Design review of the part shown in the three views and the two pictorial views. Dimensions are in mm from the part's minimum x, y and z. A direction names the side the tool comes from. Coordinates: 2 decimals unless noted, no trailing zeros. Write each loop counter-clockwise with the first axis right and the second up, starting at its lowest first coordinate (ties: lowest second). Pieces come first, ordered by that corner, then holes. Notation, with made-up numbers: (47, 32.5) - (106, 32.5) arc R32 ccw to (106, 59.5) - close; hole circle Ø5 at (26.5, 42.5). An arc over 180 degrees is marked (long way). Write each question's results on one line, items separated by ' | '.
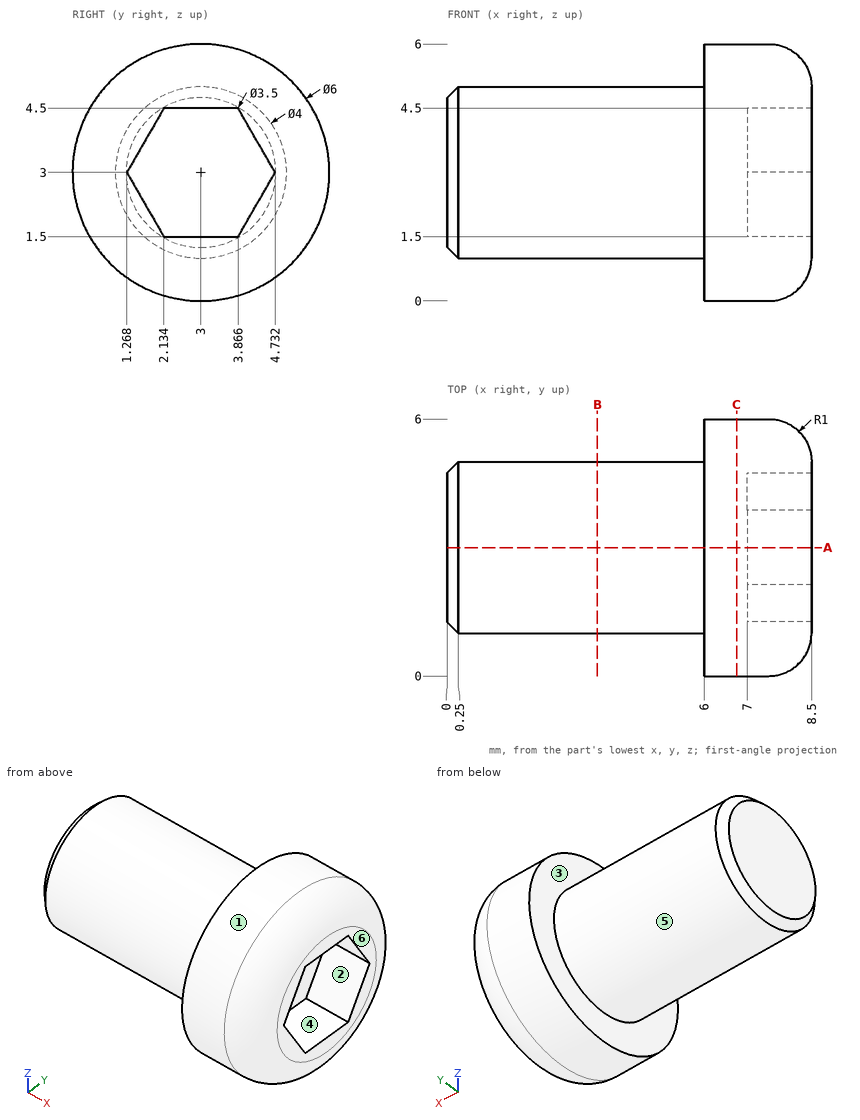
Q1. For the marked faces 1, 2 and 3, list the 3-axis set-ups (+Z, -Z, +X, -X, +Y, -Y) from which the entire face can be reached by the end or side of a thin tool; tool diameter is ignored.
Results found:
face 1: +X, -X | face 2: +X | face 3: -X
Q2. Take a section at A-A on y = 3. State the section outline as (x, z) points, plus the area to 3 significant figures.
Results found:
outline: (0, 1.25) - (0.25, 1) - (6, 1) - (6, 0) - (7.5, 0) arc R1 ccw to (8.5, 1) - (8.5, 1.5) - (7, 1.5) - (7, 4.5) - (8.5, 4.5) - (8.5, 5) arc R1 ccw to (7.5, 6) - (6, 6) - (6, 5) - (0.25, 5) - (0, 4.75) - close | area: 34.0 mm2
Q3. Wall thickness on line 1 along X through (y, z) = (2.25, 3.4); line 2 along Z through (x, y) = (3, 4); line 3 along Y through (x, z) = (8, 1.6): over which ranges is each line inside the solid? List them lowest first. Write a range as from..to.
Results found:
line 1: 0..7 | line 2: 1.27..4.73 | line 3: 0.5..2.08, 3.92..5.5
Q4. For pin 1 (0.9 mm diameter, centred on y = 3.5, z = 3, fed in from +X); pin 2 (2 mm diameter, centred on y = 3.5, z = 4, fed in from +X); pin 3 (3 mm diameter, centred on x = 4, z = 3, fed in from -Y); pin 4 (3 mm diameter, centred on x = 3, y = 1, fed in from -Z), all flat-tipped, find the tip position at first contact; note any pin that passes through.
Results found:
pin 1: x = 7 | pin 2: x = 8.5 | pin 3: y = 1 | pin 4: z = 1.06
Q5. Mouldability with a two-part tool opening along Z and no side actions: class the marked faces 4, 5 and 6 as pulls with the +Z half, pulls with the -Z half, needs draft (parallel to the pull), parting line crosses it, or undercut.
Results found:
face 4: undercut | face 5: parting line crosses it | face 6: needs draft
Q6. Take a section at C-C on x = 6.75. State the section outline as (y, z) points, plus the area to 3 significant figures.
Results found:
outline: circle Ø6 at (3, 3) | area: 28.3 mm2
Q7. Take a section at B-B on x = 3.5. State the section outline as (y, z) points.
Results found:
outline: circle Ø4 at (3, 3)
